Can you work these out from the model? Positions are in its coordinate system, mm. Round coordinates to 2 decimals unless told otherwise and drop trailing zeros. Write each loop counter-clockwise with the first axis right and the second up, starting at its lowest first coordinate (ties: lowest second). Pieces come first, ordered by that corner, then holes.
Q1. If we section it at C-C (x = 6.5): Please give me the cut outline in (y, z) (3 decimals), plus the area to 3 significant figures.
Q2. If we section it at D-D (z = 0): Please give me the cut outline in (x, y) (3 decimals).
Q3. If we section it at B-B (z = -2.25): Please give me the cut outline in (x, y) (3 decimals), plus the area to 3 significant figures.
Q4. Please list where these lines run through material, in increasing order: line 1 along Z through (x, y) = (-4.5, -13.5); line 2 along X through (y, z) = (-3, 0) (3 decimals); line 3 along Y through (x, z) = (13.5, 0.75).
Q5. If we section it at A-A (y = -8.5): Please give me the cut outline in (x, z) (3 decimals).
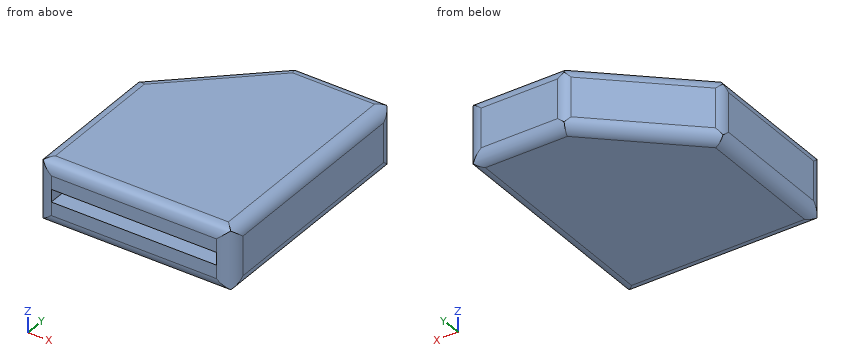
from build123d import *

# Parameters (mm, degrees)
F1_DEPTH      = 5.08
F1_DEPTH_BACK = 5.08
F2_R          = 1.905
F3_T1_DEPTH   = 19.05
F3_T3_DEPTH   = 11.9486373525
F3_T5_DEPTH   = 11.278635061
F4_W          = 26.67
F4_H          = 2.0311224633
F5_DEPTH      = 25.4


# Not quite as in the source:
# - a fillet or chamfer that OpenCascade refuses, or shapes differently, is made with other operations: its cross-section is extruded or revolved along the edge and cut away or added


with BuildPart() as f1:
    # F0 (on Top) → F1 (new body, two sides)
    with BuildSketch(Plane.XY) as f1_sk:
        Polygon((-15.875, -19.05), (15.875, -19.05), (15.875, 19.05), (0, 19.05), (-15.875, 4.5436509977), align=None)
    extrude(amount=F1_DEPTH)
    extrude(f1_sk.sketch, amount=-F1_DEPTH_BACK)

    # F2
    f2_edges = [f1.edges().sort_by_distance(p)[0] for p in [
        (-15.875, -7.253175, 5.08),
        (0, -19.05, 5.08),
        (15.875, 0, 5.08),
        (7.9375, 19.05, 5.08),
        (-7.9375, 11.796825, 5.08),
        (-15.875, -7.253175, -5.08),
        (0, -19.05, -5.08),
        (15.875, 0, -5.08),
        (7.9375, 19.05, -5.08),
        (-7.9375, 11.796825, -5.08),
    ]]
    fillet(f2_edges, radius=F2_R)

    # F3: fillet of radius 2.54 on 15 edges, made by hand

    # F3_s2 → F3_t1 (cut)
    with BuildSketch(Plane.XY.offset(-9.525)):
        with BuildLine():
            ThreePointArc((13.335, -19.05), (15.1310512242, -18.3060512242), (15.875, -16.51))
            Line((15.875, -16.51), (15.875, -19.05))
            Line((15.875, -19.05), (13.335, -19.05))
        make_face()
        with BuildLine():
            ThreePointArc((-15.875, -16.51), (-15.1310512242, -18.3060512242), (-13.335, -19.05))
            Line((-13.335, -19.05), (-15.875, -19.05))
            Line((-15.875, -19.05), (-15.875, -16.51))
        make_face()
        with BuildLine():
            ThreePointArc((13.335, 19.05), (15.1310512242, 18.3060512242), (15.875, 16.51))
            Line((15.875, 16.51), (15.875, 19.05))
            Line((15.875, 19.05), (13.335, 19.05))
        make_face()
    extrude(amount=F3_T1_DEPTH, mode=Mode.SUBTRACT)

    # F3_s4 → F3_t3 (cut)
    with BuildSketch(Plane.XY.offset(-5.9743186762)):
        with BuildLine():
            ThreePointArc((-15.875, 3.4239235272), (-15.6591819915, 4.4485103076), (-15.048403094, 5.2989834829))
            Line((-15.048403094, 5.2989834829), (-15.875, 4.5436509977))
            Line((-15.875, 4.5436509977), (-15.875, 3.4239235272))
        make_face()
    extrude(amount=F3_T3_DEPTH, mode=Mode.SUBTRACT)

    # F3_s6 → F3_t5 (cut)
    with BuildSketch(Plane.XY.offset(-5.6393175305)):
        with BuildLine():
            ThreePointArc((-0.7276760818, 18.3850599557), (0.0667744257, 18.8779371072), (0.9857270122, 19.05))
            Line((0.9857270122, 19.05), (0, 19.05))
            Line((0, 19.05), (-0.7276760818, 18.3850599557))
        make_face()
    extrude(amount=F3_T5_DEPTH, mode=Mode.SUBTRACT)

    # F4 (on face) → F5 (cut)
    with BuildSketch(Plane.XZ.offset(19.05)):
        Rectangle(F4_W, F4_H)
    extrude(amount=-F5_DEPTH, mode=Mode.SUBTRACT)


solid = f1.part
A:
1. outline: (-19.05, -3.175) arc R1.905 ccw to (-17.145, -5.08) - (17.145, -5.08) arc R1.905 ccw to (19.05, -3.175) - (19.05, 3.175) arc R1.905 ccw to (17.145, 5.08) - (-17.145, 5.08) arc R1.905 ccw to (-19.05, 3.175) - (-19.05, 1.016) - (6.35, 1.016) - (6.35, -1.016) - (-19.05, -1.016) - close
1. area: 332 mm2
2. outline: (-15.875, -16.51) arc R2.54 ccw to (-13.335, -19.05) - (-13.335, 6.35) - (13.335, 6.35) - (13.335, -19.05) arc R2.54 ccw to (15.875, -16.51) - (15.875, 16.51) arc R2.54 ccw to (13.335, 19.05) - (0.986, 19.05) arc R2.54 ccw to (-0.728, 18.385) - (-15.048, 5.299) arc R2.54 ccw to (-15.875, 3.424) - close
3. outline: (-15.875, -16.51) arc R2.54 ccw to (-13.335, -19.05) - (13.335, -19.05) arc R2.54 ccw to (15.875, -16.51) - (15.875, 16.51) arc R2.54 ccw to (13.335, 19.05) - (0.986, 19.05) arc R2.54 ccw to (-0.728, 18.385) - (-15.048, 5.299) arc R2.54 ccw to (-15.875, 3.424) - close
3. area: 1,090 mm2
4. line 1: z = -5.08 to -1.02, 1.02 to 5.08
4. line 2: x = -15.875 to -13.335, 13.335 to 15.875
4. line 3: y = -19.04 to 19.04
5. outline: (-15.875, -3.175) arc R1.905 ccw to (-13.97, -5.08) - (13.97, -5.08) arc R1.905 ccw to (15.875, -3.175) - (15.875, 3.175) arc R1.905 ccw to (13.97, 5.08) - (-13.97, 5.08) arc R1.905 ccw to (-15.875, 3.175) - close; hole (-13.335, -1.016) - (13.335, -1.016) - (13.335, 1.016) - (-13.335, 1.016) - close
